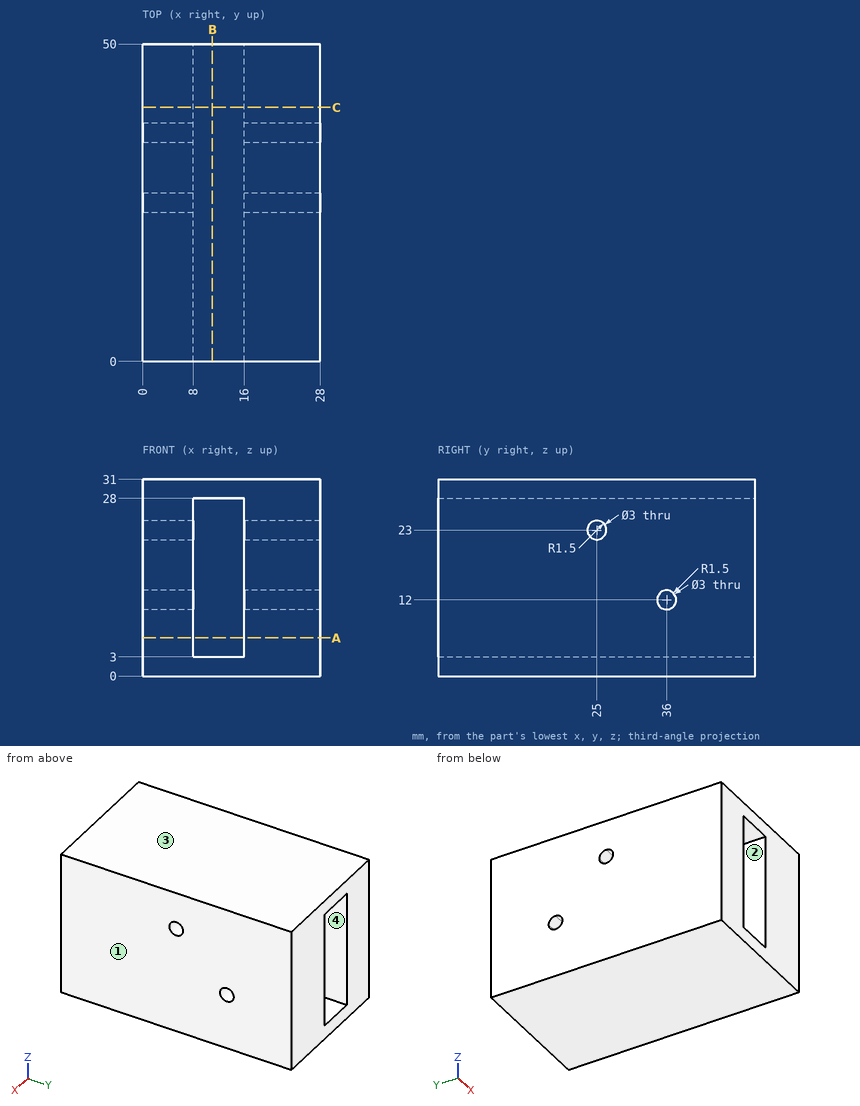
Geometry check sheet. Reference: drawing and pictorial views, mm from the part's lowest x, y, z. Round coordinates to 2 decimals unless told otherwise and drop trailing zeros. Order: outer loops, then holes, each group sorted by start corner. A loop starts at its lowest first (then second) coordinate and runs counter-clockwise, first axis right, second up. Notation, with made-up numbers: (44, 40) - (90, 40) arc R28 ccw to (90, 63) - close; hole circle Ø11 at (78.5, 27.25). An arc over 180 degrees is marked (long way). Use a Markdown table: item, result. Add a question column.
1) Section check A-A (z = 6). Record the cut outline in (x, y).
2) Section check B-B (x = 11). Record the cut outline in (y, z), then the cut area to 3 significant figures.
3) Mould release check, pull along X, two halves, no side actions. Record for the marked faces 1, 2, 3 and 4: released by +X, released by -X, zero draft, split by the parting line, or undercut.
4) Section check C-C (y = 40). Record the cut outline in (x, z), then the cut area to 3 significant figures.
5) Thickness scan on line 1 along Z through (x, y) = (24.75, 25); line 2 along X through (y, z) = (21.5, 5); line 3 along Z through (x, y) = (5.5, 36). Record the ranges inside material, lowest first.
Established:
| question | item | result |
|---|---|---|
| 1 | outline | (0, 0) - (8, 0) - (8, 50) - (0, 50) - close; (16, 0) - (28, 0) - (28, 50) - (16, 50) - close |
| 2 | outline | (0, 0) - (50, 0) - (50, 3) - (0, 3) - close; (0, 28) - (50, 28) - (50, 31) - (0, 31) - close |
| 2 | area | 300 mm2 |
| 3 | face 1 | released by +X |
| 3 | face 2 | undercut |
| 3 | face 3 | zero draft |
| 3 | face 4 | undercut |
| 4 | outline | (0, 0) - (28, 0) - (28, 31) - (0, 31) - close; hole (8, 3) - (16, 3) - (16, 28) - (8, 28) - close |
| 4 | area | 668 mm2 |
| 5 | line 1 | 0 to 21.5, 24.5 to 31 |
| 5 | line 2 | 0 to 8, 16 to 28 |
| 5 | line 3 | 0 to 10.5, 13.5 to 31 |
